Autodesk Inventor part; units mm, degrees
sketch "スケッチ1" plane through (0, 0, 0) normal (0, 0, 1) x (1, 0, 0)
  circle A0 centre (0, 0) radius 15
  dimension "d0" = 30
extrude "押し出し1" add sketch "スケッチ1" along normal blind 22.5
sketch "スケッチ2" plane through (0, 0, 22.5) normal (0, 0, 1) x (1, 0, 0)
  circle A0 centre (0, 0) radius 10
  dimension "d3" = 20
extrude "押し出し2" add sketch "スケッチ2" along normal blind 22.5
ref_plane "作業平面1" through (0, 15, 0) normal (0, 1, 0) x (-1, 0, 0)
sketch "スケッチ3" plane through (0, 15, 0) normal (0, 1, 0) x (-1, 0, 0)
  line L0 (0, 0) -> (0, 20)
  line L1 (0, 20) -> (0, 16)
  arc A0 (4, 16) -> (0, 20) centre (0, 16) ccw
  arc A1 (0, 20) -> (-4, 16) centre (0, 16) ccw
  line L2 (4, 16) -> (4, 0)
  line L3 (-4, 16) -> (-4, 0)
  line L4 (4, 0) -> (-4, 0)
  dimension "d7" = 20
  dimension "d8" = 4
extrude "押し出し3" cut sketch "スケッチ3" against normal blind 4
mirror "ミラー1" about plane through (0, 0, 0) normal (0, 0, 1) of "押し出し1", "押し出し2", "押し出し3"
properties part number "shaft1"
Design review of the part built by this model. Coordinates are the model's own, in mm. A direction names the side the tool comes from. Give positions to 0.01 mm unless a question says otherwise; leave off trailing zeros. Order: outer loops, then holes, each group sorted by start corner. A loop starts at its lowest first (then second) coordinate and runs counter-clockwise, first axis right, second up. Notation, with made-up numbers: (84.5, 76) -> (129.5, 76) arc R24 ccw to (129.5, 94) -> close; hole circle Ø1 at (71, 68). An arc over 180 degrees is marked (long way). Write each question's results on one line, items separated by ' | '. Start each with the question number.
Q1. Add section A-A on x = 0. Give the boundary of the cut face in (y, z).
Q2. Add section D-D on z = -31. Give the boundary of the cut face in (x, y).
Q3. Wall thickness on L1, parallel to Z at x = -11.5, y = 6.5; L2, parallel to X at y = 12, z = 5; L3, parallel to Y at x = -0.5, z = 3.5: over which ranges is each line inside the solid? List them lowest first. Write a range as from..to.
Q4. For pin 1 (1 mm diameter, centred on x = -4, y = -12, fed in from +Z); pin 2 (5 mm diameter, centred on x = 8, z = -1, fed in from +Y); pin 3 (12 mm diameter, centred on y = -8, z = -3.5, fed in from -X), all flat-tipped, find the tip position at first contact; note any pin that passes through.
Q5. Add section B-B on y = 12. Give the boundary of the cut face in (x, z).
Q6. Mouldability with a two-part tool opening along Z and no side actions: class faces 4 (the cylindrical face through (0, 13, -20)), 5 (the cylindrical face through (-2.17, 9.76, 33.59)), 6 (the flat face through (-4, 13, 0)), 7 (the flat face through (3, -10, 22.5)) as +Z half, -Z half, draft (parallel to the pull), parting line (faces both ways), or undercut.
Q7. Add section C-C on y = 0. Give the boundary of the cut face in (x, z), and give its area (3 significant figures).
Q8. Machinability: for faces 1 (the flat face through (0, 11, 0)), 2 (the flat face through (0, 0, -45)), 3 (the cylindrical face through (-2.17, -9.76, -33.59)), which of the approach directions +Z, -Z, +X, -X, +Y, -Y give a long, thin tool a straight path to every point of the face, cutting with its end or side? Answer none if there is none.
Found:
1) outline: (-15, -22.5) -> (-10, -22.5) -> (-10, -45) -> (10, -45) -> (10, -22.5) -> (15, -22.5) -> (15, -20) -> (11, -20) -> (11, 20) -> (15, 20) -> (15, 22.5) -> (10, 22.5) -> (10, 45) -> (-10, 45) -> (-10, 22.5) -> (-15, 22.5) -> close
2) outline: circle Ø20 at (0, 0)
3) L1: z = -22.5..22.5 | L2: x = -9..-4, 4..9 | L3: y = -14.99..11
4) pin 1: stops at z = 22.5 | pin 2: stops at y = 13.96 | pin 3: stops at x = -14.87
5) outline: (-9, -22.5) -> (9, -22.5) -> (9, 22.5) -> (-9, 22.5) -> close; hole (-4, -16) arc R4 ccw to (4, -16) -> (4, 16) arc R4 ccw to (-4, 16) -> close
6) face 4: undercut | face 5: draft | face 6: undercut | face 7: +Z half
7) outline: (-15, -22.5) -> (-10, -22.5) -> (-10, -45) -> (10, -45) -> (10, -22.5) -> (15, -22.5) -> (15, 22.5) -> (10, 22.5) -> (10, 45) -> (-10, 45) -> (-10, 22.5) -> (-15, 22.5) -> close | area: 2,250 mm2
8) face 1: +Y | face 2: -Z, +X, -X, +Y, -Y | face 3: -Z
